For this review, take the finished solid that the model builds, in its own axes (mm). Face numbers are marked on the shaded views. A direction names the side the tool comes from. Coordinates: 2 decimals unless noted, no trailing zeros. Loops run counter-clockwise (first coordinate to the right, second up) from the corner with the lowest first, then second, coordinate; pieces in that order, holes last. Notation, with made-up numbers: (70, -21.5) -> (102, -21.5) arc R14 ccw to (102, -12.5) -> close; hole circle Ø4 at (-16, 11.25). An arc over 180 degrees is marked (long way). Use a Markdown table: item, result.
from build123d import *

# Parameters (mm, degrees)
F0_W     = 101.6
F0_H     = 63.5
F1_DEPTH = 38.1
F2_W     = 50.8
F2_H     = 25.4
F3_DEPTH = 38.101
F4_W     = 76.2
F4_H     = 63.5
F5_DEPTH = 25.4


with BuildPart() as f1:
    # F0 (on Front) → F1 (new body)
    with BuildSketch(Plane.XZ):
        Rectangle(F0_W, F0_H)
    extrude(amount=F1_DEPTH)

    # F2 (on face) → F3 (cut, through all)
    with BuildSketch(Plane.XZ.offset(38.1)):
        with Locations((25.4, 0)):
            Rectangle(F2_W, F2_H)
    extrude(amount=-F3_DEPTH, mode=Mode.SUBTRACT)

    # F4 (on face) → F5 (cut)
    with BuildSketch(Plane.XZ.offset(38.1)):
        with Locations((12.7, 0)):
            Rectangle(F4_W, F4_H)
    extrude(amount=-F5_DEPTH, mode=Mode.SUBTRACT)


solid = f1.part
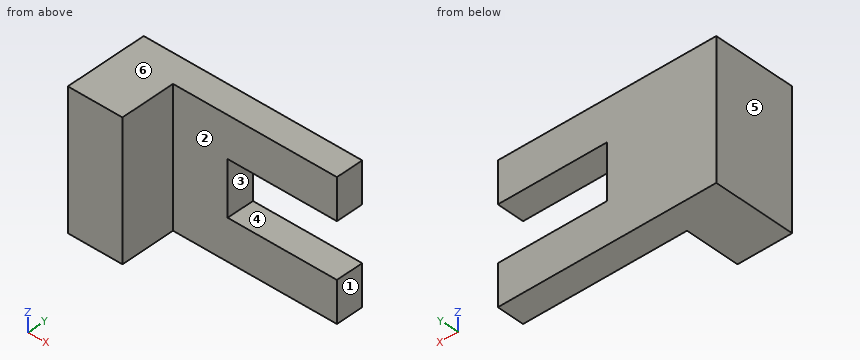
(1) Take a section at C-C on z = -18. Write out the cut boundary in (x, y).
Found:
| item | result |
|---|---|
| outline | (-50.8, -38.1) -> (-25.4, -38.1) -> (-25.4, -12.7) -> (50.8, -12.7) -> (50.8, 0) -> (-50.8, 0) -> close |
(2) Take a section at D-D on z = -4.5. Write out the cut boundary in (x, y).
Found:
| item | result |
|---|---|
| outline | (-50.8, -38.1) -> (-25.4, -38.1) -> (-25.4, -12.7) -> (0, -12.7) -> (0, 0) -> (-50.8, 0) -> close |
(3) For line 1 along Z through (x, y) = (24, -7); line 2 along X through (y, z) = (-24, 25.5); line 3 along Y through (x, z) = (3, 29), list the stretches that pass through material, from the lowest coordinate up.
Found:
| item | result |
|---|---|
| line 1 | z = -31.75 to -12.7, 12.7 to 31.75 |
| line 2 | x = -50.8 to -25.4 |
| line 3 | y = -12.7 to 0 |
(4) Mouldability with a two-part tool opening along Z and no side actions: class the marked faces 4, 5 and 6 as pulls with the +Z half, pulls with the -Z half, needs draft (parallel to the pull), parting line crosses it, or undercut.
Found:
| item | result |
|---|---|
| face 4 | undercut |
| face 5 | needs draft |
| face 6 | pulls with the +Z half |
(5) For the marked faces 1, 2 and 3, list the 3-axis set-ups (+Z, -Z, +X, -X, +Y, -Y) from which the entire face can be reached by the end or side of a thin tool; tool diameter is ignored.
Found:
| item | result |
|---|---|
| face 1 | +Z, -Z, +X, +Y, -Y |
| face 2 | +Z, -Z, +X, -Y |
| face 3 | +X, +Y, -Y |
(6) For pin 1 Ø6 at (x, z) = (-15, -19.5) entering from +Y; pin 2 Ø5 at (y, z) = (-28, 5.5) entering from +X; pin 3 Ø8 at (x, z) = (18, 17.5) entering from -Y; pin 4 Ø10 at (y, z) = (-5, 5) entering from +X, all flat-tipped, find the tip position at first contact; note any pin that passes through.
Found:
| item | result |
|---|---|
| pin 1 | stops at y = 0 |
| pin 2 | stops at x = -25.4 |
| pin 3 | stops at y = -12.7 |
| pin 4 | stops at x = 0 |
(7) Take a section at B-B on y = -7. Write out the cut boundary in (x, z), plus the area to 3 significant figures.
Found:
| item | result |
|---|---|
| outline | (-50.8, -31.75) -> (50.8, -31.75) -> (50.8, -12.7) -> (0, -12.7) -> (0, 12.7) -> (50.8, 12.7) -> (50.8, 31.75) -> (-50.8, 31.75) -> close |
| area | 5,160 mm^2 |
(8) Take a section at A-A on x = 2.5. Write out the cut boundary in (y, z), plus the area to 3 significant figures.
Found:
| item | result |
|---|---|
| outline | (-12.7, -31.75) -> (0, -31.75) -> (0, -12.7) -> (-12.7, -12.7) -> close; (-12.7, 12.7) -> (0, 12.7) -> (0, 31.75) -> (-12.7, 31.75) -> close |
| area | 484 mm^2 |
